Geometry: see drawing. Coordinates: mm, zero at the bounding-box minimum. Coordinates: 2 decimals unless noted, no trailing zeros.
Item 1: Contact query for flat-ended pins moving along their axis: P1, Ø8, axis at x = 41.38, y = 13.5, coming from the -Z side; P2, Ø7.5, axis at x = 59.38, y = 4.5, coming from the +Z side. Output: stop coordinate, or through.
Item 2: Section A-A on z = 8.5. State how many separate pieces and enclosed holes the cut face has, then the cut area to 3 significant figures.
Item 3: Ray query, line 1 (Y direction, x = 23.38, z = 4.55); line 2 (Y direction, x = 24, z = 5.75); line 3 (Z direction, x = 20.5, y = 6). Return the intervals inside material, ascending.
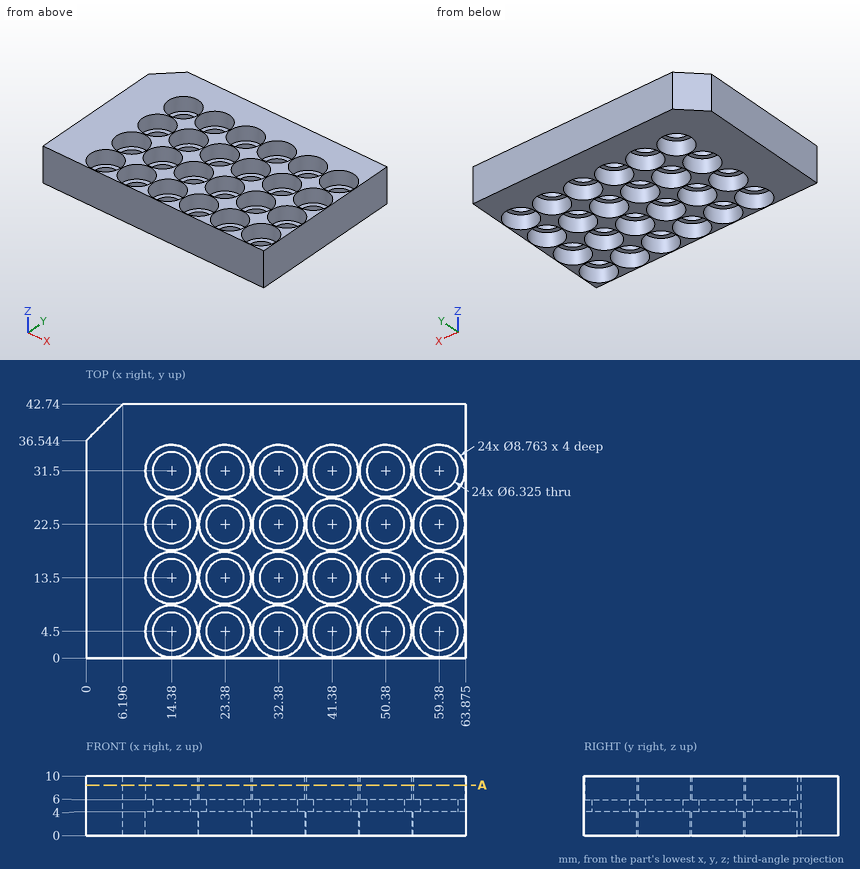
Answer list:
1. P1: stops at z = 4
1. P2: stops at z = 6
2. separate pieces: 1
2. enclosed holes: 24
2. area: 1,260 mm2
3. line 1: y = 0 to 1.34, 7.66 to 10.34, 16.66 to 19.34, 25.66 to 28.34, 34.66 to 42.74
3. line 2: y = 0 to 1.4, 7.6 to 10.4, 16.6 to 19.4, 25.6 to 28.4, 34.6 to 42.74
3. line 3: z = 4 to 6
